CAD build for the part. Positions are in the model's coordinates, mm. Face numbers are marked on the shaded views. Give positions to 0.01 mm unless a question says otherwise; leave off trailing zeros. Loops run counter-clockwise (first coordinate to the right, second up) from the corner with the lowest first, then second, coordinate; pieces in that order, holes last.
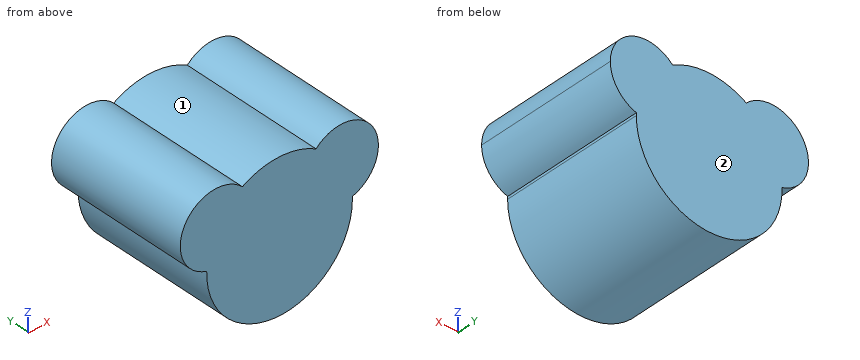
```python
from build123d import *

# Parameters (mm, degrees)
F1_DEPTH = 76.2


with BuildPart() as f1:
    # F0 (on Front) → F1 (new body)
    with BuildSketch(Plane.XZ):
        with BuildLine():
            Line((0, 0), (16.3282829281, 9.8127303346))
            ThreePointArc((16.3282829281, 9.8127303346), (13.7388791973, 21.866806576), (19.0733598326, 32.9820700487))
            ThreePointArc((19.0733598326, 32.9820700487), (-0.2140813256, 38.099398541), (-19.4427976439, 32.7656469458))
            ThreePointArc((-19.4427976439, 32.7656469458), (-15.2854652775, 26.5722258682), (-13.825048557, 19.2572371428))
            ThreePointArc((-13.825048557, 19.2572371428), (-14.4897645301, 14.2688675447), (-16.4375242785, 9.6286185714))
            Line((-16.4375242785, 9.6286185714), (0, 0))
        make_face()
        with BuildLine():
            ThreePointArc((32.6565658563, 19.6254606691), (36.5259490937, 10.8381291192), (38.0756304159, 1.3624861223))
            ThreePointArc((38.0756304159, 1.3624861223), (47.9231253878, 8.2309593606), (51.7065658563, 19.6254606691))
            ThreePointArc((51.7065658563, 19.6254606691), (39.8726044249, 37.2558687011), (19.0733598326, 32.9820700487))
            ThreePointArc((19.0733598326, 32.9820700487), (26.7132187591, 27.1664120474), (32.6565658563, 19.6254606691))
        make_face()
        with BuildLine():
            ThreePointArc((16.3282829281, 9.8127303346), (25.7569703489, 1.8688258011), (38.0756304159, 1.3624861223))
            ThreePointArc((38.0756304159, 1.3624861223), (36.5259490937, 10.8381291192), (32.6565658563, 19.6254606691))
            Line((32.6565658563, 19.6254606691), (16.3282829281, 9.8127303346))
        make_face()
        with BuildLine():
            Line((16.3282829281, 9.8127303346), (32.6565658563, 19.6254606691))
            ThreePointArc((32.6565658563, 19.6254606691), (26.7132187591, 27.1664120474), (19.0733598326, 32.9820700487))
            ThreePointArc((19.0733598326, 32.9820700487), (13.7388791973, 21.866806576), (16.3282829281, 9.8127303346))
        make_face()
        with BuildLine():
            ThreePointArc((-38.0885373309, 0.934518054), (-0.4672941756, -38.0971342249), (38.1, 0))
            ThreePointArc((38.1, 0), (38.0939071168, 0.6813520217), (38.0756304159, 1.3624861223))
            ThreePointArc((38.0756304159, 1.3624861223), (25.7569703489, 1.8688258011), (16.3282829281, 9.8127303346))
            Line((16.3282829281, 9.8127303346), (0, 0))
            Line((0, 0), (-16.4375242785, 9.6286185714))
            ThreePointArc((-16.4375242785, 9.6286185714), (-25.7763452104, 1.5792590119), (-38.0885373309, 0.934518054))
        make_face()
        with BuildLine():
            ThreePointArc((-19.4427976439, 32.7656469458), (-49.3125728356, 28.8858557141), (-38.0885373309, 0.934518054))
            ThreePointArc((-38.0885373309, 0.934518054), (-36.6454381775, 10.4269775477), (-32.875048557, 19.2572371428))
            ThreePointArc((-32.875048557, 19.2572371428), (-27.0168196061, 26.8645018262), (-19.4427976439, 32.7656469458))
        make_face()
        with BuildLine():
            ThreePointArc((-32.875048557, 19.2572371428), (-36.6454381775, 10.4269775477), (-38.0885373309, 0.934518054))
            ThreePointArc((-38.0885373309, 0.934518054), (-25.7763452104, 1.5792590119), (-16.4375242785, 9.6286185714))
            Line((-16.4375242785, 9.6286185714), (-32.875048557, 19.2572371428))
        make_face()
        with BuildLine():
            ThreePointArc((-19.4427976439, 32.7656469458), (-27.0168196061, 26.8645018262), (-32.875048557, 19.2572371428))
            Line((-32.875048557, 19.2572371428), (-16.4375242785, 9.6286185714))
            ThreePointArc((-16.4375242785, 9.6286185714), (-14.4897645301, 14.2688675447), (-13.825048557, 19.2572371428))
            ThreePointArc((-13.825048557, 19.2572371428), (-15.2854652775, 26.5722258682), (-19.4427976439, 32.7656469458))
        make_face()
    extrude(amount=F1_DEPTH)


solid = f1.part
```
1. Probe line 1 along X through (y, z) = (-47.5, -0.5); line 2 along Z through (x, y) = (-39, -29.5); line 3 along Z through (x, y) = (31.5, -19). List the from-to ranges inside material, lowest first.
Responses:
line 1: x = -38.1 to 38.1
line 2: z = 1.22 to 37.3
line 3: z = -21.43 to 38.64
2. Pull direction X, two halves, no side cores. Call the marked faces 1 and 2: released by +X, released by -X, zero draft, split by the parting line, or undercut.
Responses:
face 1: undercut
face 2: zero draft
3. Saw through at C-C, the plane z = -19.5. List the corners of the cut face in (x, y).
Responses:
outline: (-32.73, -76.2) - (32.73, -76.2) - (32.73, 0) - (-32.73, 0) - close
4. Drop flat-ended pins along their axis: pin 1 (8 mm diameter, centred on x = 32, y = -38, fed in from -Z); pin 2 (6 mm diameter, centred on y = -31.5, z = 3.5, fed in from +X); pin 3 (8 mm diameter, centred on x = -14, y = -32.5, fed in from -Z). Give the stop position or say it passes through.
Responses:
pin 1: stops at z = -25.84
pin 2: stops at x = 46.46
pin 3: stops at z = -36.76
5. Saw through at A-A, the plane x = 13.5. List the corners of the cut face in (y, z), and give its area (3 significant figures).
Responses:
outline: (-76.2, -35.63) - (0, -35.63) - (0, 35.63) - (-76.2, 35.63) - close
area: 5,430 mm2
6. Saw through at B-B, the plane y = -40. List the corners of the cut face in (x, z).
Responses:
outline: (-38.09, 0.93) arc R38.1 ccw (long way) to (38.08, 1.36) arc R19.05 ccw (long way) to (19.07, 32.98) arc R38.1 ccw to (-19.44, 32.77) arc R19.05 ccw (long way) to start
